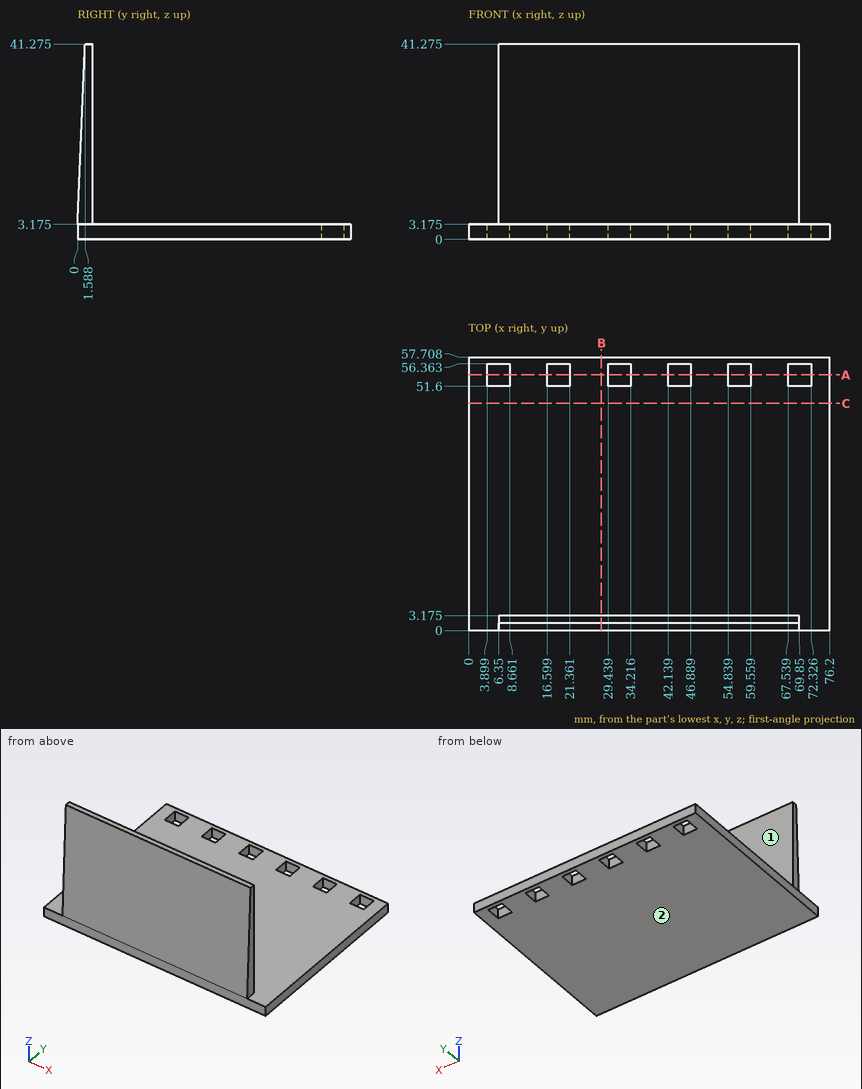
For this review, use the dimensioned drawing (mm, ordinates from the lowest corner) and the shaded views. A direction names the side the tool comes from. Round coordinates to 2 decimals unless told otherwise and drop trailing zeros. Order: outer loops, then holes, each group sorted by start corner. A loop starts at its lowest first (then second) coordinate and runs counter-clockwise, first axis right, second up. Notation, with made-up numbers: (28, -16) -> (74, -16) arc R12 cw to (74, -5) -> close; hole circle Ø1 at (-23.5, 75). An arc over 180 degrees is marked (long way). Write item = value, one per line. Start each with the question number.
Item 1: Clearance check with flat-ended pins moving along their axes: pin 1 Ø12 at (x, y) = (58.5, 25.5) entering from +Z (1 decimal); pin 2 Ø2.5 at (y, z) = (2, 29.5) entering from -X; pin 3 Ø1.6 at (y, z) = (53.5, 2.5) entering from -X; pin 4 Ø1.6 at (y, z) = (2.5, 15.5) entering from +X. State where each tip first meets the part, or that it passes through.
Item 2: For the marked faces 1 and 2, list the 3-axis set-ups (+Z, -Z, +X, -X, +Y, -Y) from which the entire face can be reached by the end or side of a thin tool; tool diameter is ignored.
Item 3: Consider section A-A on y = 54. Write out the cut boundary in (x, z) (1 decimal).
Item 4: For line 1 along Z through (x, y) = (30.5, 30.5) (1 decimal); line 2 along X through (y, z) = (3, 23.5); line 3 along Y through (x, z) = (57, 18) (1 decimal), list the stretches that pass through material, from the lowest coordinate up.
Item 5: Consider section B-B on x = 28. Write out the cut boundary in (y, z) (1 decimal).
Item 6: Consider section C-C on y = 48. Write out the cut boundary in (x, z) (1 decimal), plus the area to 3 significant figures.
Conclusion:
q1.pin_1 = 3.2
q1.pin_2 = 6.35
q1.pin_3 = 0
q1.pin_4 = 69.85
q2.face_1 = +Z, +X, -X, +Y
q2.face_2 = -Z, +X, -X, +Y, -Y
q3.outline = (0, 0) -> (3.9, 0) -> (3.9, 3.2) -> (0, 3.2) -> close; (8.7, 0) -> (16.6, 0) -> (16.6, 3.2) -> (8.7, 3.2) -> close; (21.4, 0) -> (29.4, 0) -> (29.4, 3.2) -> (21.4, 3.2) -> close; (34.2, 0) -> (42.1, 0) -> (42.1, 3.2) -> (34.2, 3.2) -> close; (46.9, 0) -> (54.8, 0) -> (54.8, 3.2) -> (46.9, 3.2) -> close; (59.6, 0) -> (67.5, 0) -> (67.5, 3.2) -> (59.6, 3.2) -> close; (72.3, 0) -> (76.2, 0) -> (76.2, 3.2) -> (72.3, 3.2) -> close
q4.line_1 = 0 to 3.2
q4.line_2 = 6.35 to 69.85
q4.line_3 = 0.6 to 3.2
q5.outline = (0, 0) -> (57.7, 0) -> (57.7, 3.2) -> (3.2, 3.2) -> (3.2, 41.3) -> (1.6, 41.3) -> (0, 3.2) -> close
q6.outline = (0, 0) -> (76.2, 0) -> (76.2, 3.2) -> (0, 3.2) -> close
q6.area = 242 mm2
